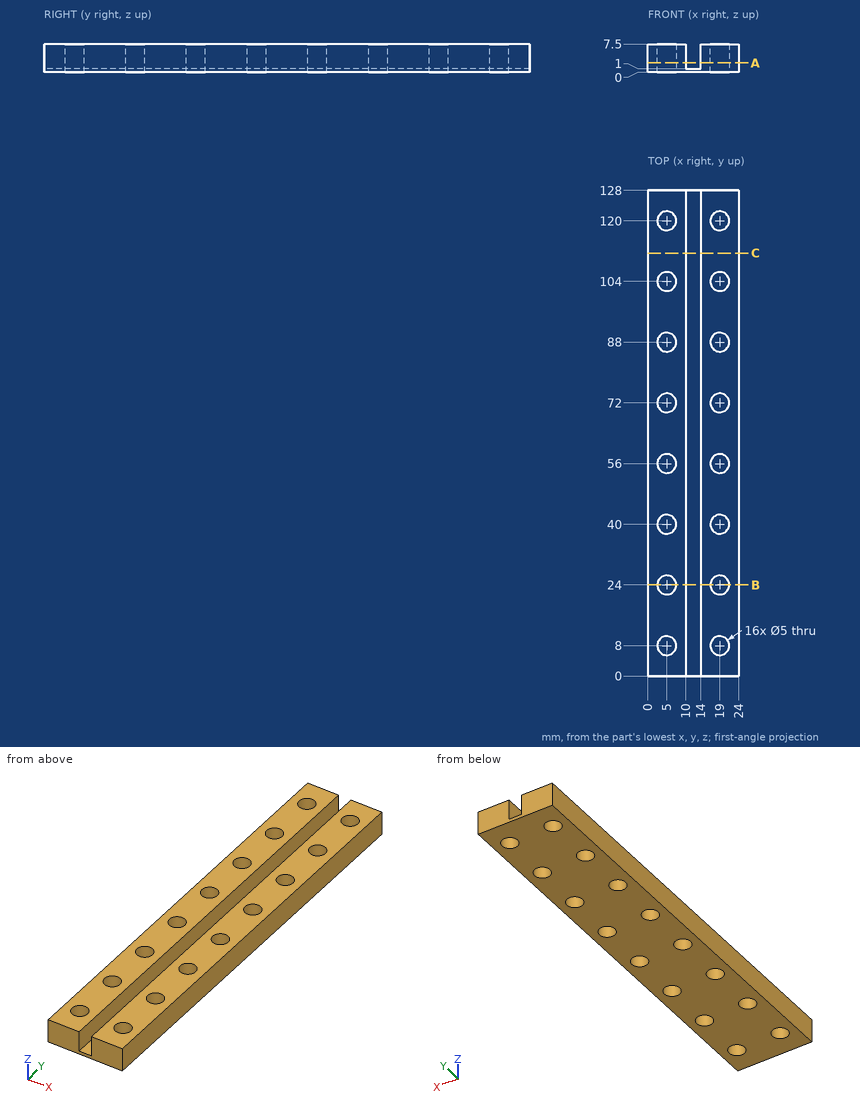
Job drawing, mm, ordinate dimensions from the low corner. One solid piece. Give positions to 0.01 mm unless a question says otherwise; leave off trailing zeros. Write each loop counter-clockwise with the first axis right and the second up, starting at its lowest first coordinate (ties: lowest second). Pieces come first, ordered by that corner, then holes. Notation, with made-up numbers: M -17.5,-18 L 17.5,-18 A26 ccw 17.5,7 Z; hole C 56.25,61.5 d11. An arc over 180 degrees is marked long. Put each result on its own line as item: value. Start each with the question number.
(1) Flat gauge pins, fed straight in: pin 1 Ø2 at (x, y) = (15, 31.5) entering from -Z; pin 2 Ø1.2 at (x, y) = (13, 34) entering from +Z. Where does each tip first touch, or does it go through?
(2) Band-saw the part on A-A, the plane z = 2.5. Give the number of separate pieces and of enclosed holes in the cut face, and give its area (3 significant figures).
(3) Band-saw the part on B-B, the plane y = 24. Write the cut outline in (x, z).
(4) Band-saw the part on C-C, the plane y = 111.5. Write the cut outline in (x, z), and give its area (3 significant figures).
(5) Probe L1, parallel to X at y = 40, z = 2; L2, parallel to X at y = 91, z = 6.25; L3, parallel to X at y = 55.5, z = 5. List the from-to ranges inside material, lowest first.
Response values:
1. pin 1: stops at z = 0
1. pin 2: stops at z = 1
2. separate pieces: 2
2. enclosed holes: 16
2. area: 2,250 mm2
3. outline: M 0,0 L 2.5,0 L 2.5,7.5 L 0,7.5 Z; M 7.5,0 L 16.5,0 L 16.5,7.5 L 14,7.5 L 14,1 L 10,1 L 10,7.5 L 7.5,7.5 Z; M 21.5,0 L 24,0 L 24,7.5 L 21.5,7.5 Z
4. outline: M 0,0 L 24,0 L 24,7.5 L 14,7.5 L 14,1 L 10,1 L 10,7.5 L 0,7.5 Z
4. area: 154 mm2
5. L1: x = 0 to 2.5, 7.5 to 10, 14 to 16.5, 21.5 to 24
5. L2: x = 0 to 10, 14 to 24
5. L3: x = 0 to 2.55, 7.45 to 10, 14 to 16.55, 21.45 to 24
